from build123d import *

# Parameters (mm, degrees)
F0_W     = 596.9
F0_H     = 152.4
F1_DEPTH = 6.35
F2_W     = 3.175
F2_H     = 3.175
F3_DEPTH = 596.901
F4_W     = 3.175
F4_H     = 3.175
F5_DEPTH = 152.4


with BuildPart() as f1:
    # F0 (on Front) → F1 (new body)
    with BuildSketch(Plane.XZ):
        Rectangle(F0_W, F0_H)
    extrude(amount=F1_DEPTH)

    # F2 (on face) → F3 (cut, through all)
    with BuildSketch(Plane.YZ.offset(298.45)):
        with Locations((-4.7625, -74.6125)):
            Rectangle(F2_W, F2_H)
        with Locations((-4.7625, 74.6125)):
            Rectangle(F2_W, F2_H)
    extrude(amount=-F3_DEPTH, mode=Mode.SUBTRACT)

    # F4 (on face) → F5 (join, through all)
    with BuildSketch(Plane.XY.offset(76.2)):
        with Locations((-300.0375, -1.5875)):
            Rectangle(F4_W, F4_H)
        with Locations((300.0375, -1.5875)):
            Rectangle(F4_W, F4_H)
    extrude(amount=-F5_DEPTH)


solid = f1.part
Read the model definition and answer for the solid it produces. Units are mm, in the model's axes. Coordinates: 2 decimals unless noted, no trailing zeros. Order: outer loops, then holes, each group sorted by start corner. A loop starts at its lowest first (then second) coordinate and runs counter-clockwise, first axis right, second up. Notation, with made-up numbers: M -11.75,75 L 8.25,75 A11 cw 8.25,90 Z; hole C 73,82 d3. An arc over 180 degrees is marked long. Put each result on its own line as item: value. Start each with the question number.
Item 1: Section A-A, the plane x = 3 is taken. Determine the outline of the cut face in (y, z) (3 decimals).
Item 2: Given pin 1 Ø2.5 at (y, z) = (-4.5, 19.5) entering from -X; pin 2 Ø1.6 at (x, y) = (127, -4.5) entering from -Z (3 decimals), each flat-ended and moving along its own axis, determine where each tip first touches the part or whether it passes through.
Item 3: Section B-B, the plane y = -5 is taken. Determine the outline of the cut face in (x, z) (3 decimals).
Item 4: Consider probe 1 along Z at (x, y) = (105, -4.5) (3 decimals); probe 2 along X at (y, z) = (-4.5, 69). Determine where each line is inside the solid, lowest interval first. Write a range as [from, to].
Computed:
1. outline: M -6.35,-73.025 L -3.175,-73.025 L -3.175,-76.2 L 0,-76.2 L 0,76.2 L -3.175,76.2 L -3.175,73.025 L -6.35,73.025 Z
2. pin 1: stops at x = -298.45
2. pin 2: stops at z = -73.025
3. outline: M -298.45,-73.025 L 298.45,-73.025 L 298.45,73.025 L -298.45,73.025 Z
4. probe 1: z = [-73.025, 73.025]
4. probe 2: x = [-298.45, 298.45]
